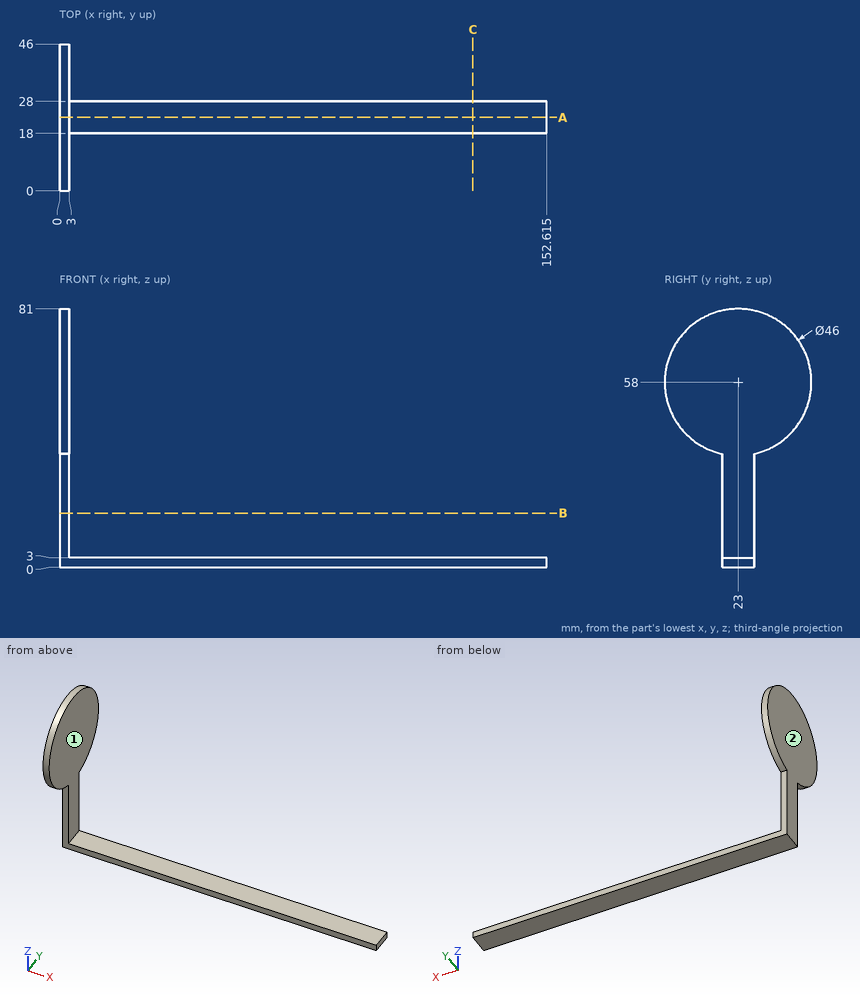
The drawing under review shows one solid part. Ordinate dimensions are in mm from its lowest x, y, z. A direction names the side the tool comes from. Coordinates: 2 decimals unless noted, no trailing zeros. Write each loop counter-clockwise with the first axis right and the second up, starting at its lowest first coordinate (ties: lowest second). Pieces come first, ordered by that corner, then holes.
1) To check wall thickness, follow L1, parallel to X at y = 40, z = 43.5. State the ranges of the line that lie inside material, in increasing order.
2) Add section C-C (x = 129.5). Write out the cut boundary in (y, z).
3) Add section A-A (y = 23). Write out the cut boundary in (x, z) (3 decimals), plus the area to 3 significant figures.
4) Add section B-B (z = 17). Write out the cut boundary in (x, y).
5) Insertion check: pin 1 (5 mm diameter, centred on y = 15, z = 31, fed in from -X); pin 2 (12 mm diameter, centred on x = 21, y = 29.5, fed in from +Z); pin 3 (1.5 mm diameter, centred on y = 13, z = 51, fed in from +X). Each pin has a flat end and moves straight along its axis. Give the tip position at first contact, or say it passes through.
6) Machinability: for the marked faces 1 and 2, which of the approach directions +Z, -Z, +X, -X, +Y, -Y give a long, thin tool a straight path to every point of the face, cutting with its end or side? Answer none if there is none.
Check result:
1. L1: x = 0 to 3
2. outline: (18, 0) - (28, 0) - (28, 3) - (18, 3) - close
3. outline: (0, 0) - (152.615, 0) - (152.615, 3) - (3, 3) - (3, 81) - (0, 81) - close
3. area: 692 mm2
4. outline: (0, 18) - (3, 18) - (3, 28) - (0, 28) - close
5. pin 1: passes through
5. pin 2: stops at z = 3
5. pin 3: stops at x = 3
6. face 1: +Z, +X, +Y, -Y
6. face 2: +Z, -Z, -X, +Y, -Y
